Here's the drawing with two shaded views (mm, measured from the low corner). I have some questions. A direction names the side the tool comes from. Coordinates: 2 decimals unless noted, no trailing zeros. Write each loop counter-clockwise with the first axis right and the second up, starting at its lowest first coordinate (ties: lowest second). Pieces come first, ordered by that corner, then holes.
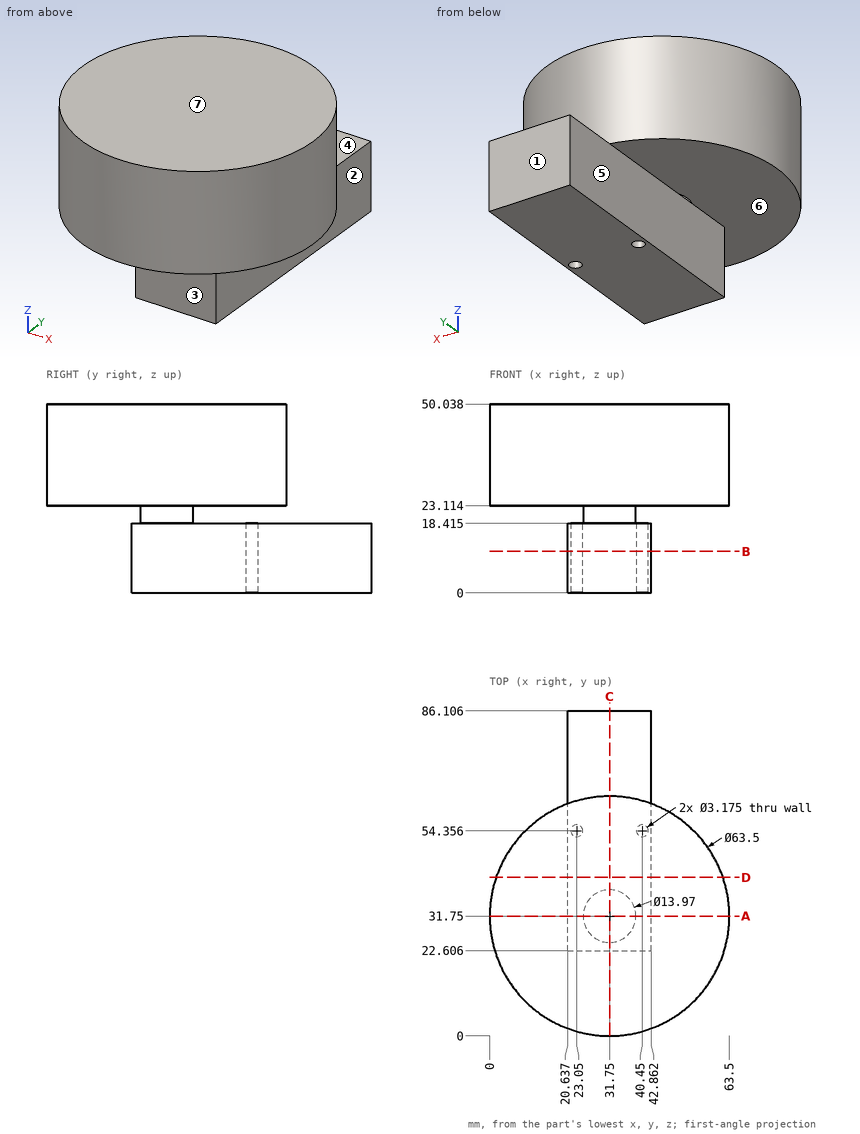
Item 1: I want a section at A-A, the plane y = 31.75. List the corners of the cut face in (x, z) for me (1 decimal), then the cut area to 3 significant figures.
Item 2: If I drill on line 1 along X through (y, z) = (54.5, 17); line 2 along Z through (x, y) = (29, 57) (1 decimal); line 3 along Z through (x, y) = (33, 66) (1 decimal), over which ranges is the centre line in solid material (lowest first)?
Item 3: Will these pins go through, and if not, where does the flat tip stop? pin 1 Ø4 at (x, z) = (54.5, 24.5) entering from -Y; pin 2 Ø9 at (y, z) = (54, 5.5) entering from +X; pin 3 Ø5.5 at (y, z) = (59, 7.5) entering from -X.
Item 4: Which directions (+Z, -Z, +X, -X, +Y, -Y) give clear straight access to the entire face, cutting with the end or side of a thin tool? Please do the marked faces 1, 2 and 3.
Item 5: I want a section at C-C, the plane x = 31.75. List the corners of the cut face in (y, z) for me (1 decimal).
Item 6: I want a section at B-B, the plane z = 11. Count the separate pieces of the cut face and the enclosed holes in it, then the cut area to 3 significant figures.
Item 7: If we mould it in two halves opening along Z, with no side actions, what happens to the marked faces 4, 5, 6 and 7? For each: released by +Z, released by -Z, zero draft, split by the parting line, or undercut.
Item 8: I want a section at D-D, the plane y = 42. List the corners of the cut face in (x, z) for me (1 decimal).
Taken from the geometry:
1. outline: (0, 23.1) - (24.8, 23.1) - (24.8, 18.4) - (20.6, 18.4) - (20.6, 0) - (42.9, 0) - (42.9, 18.4) - (38.7, 18.4) - (38.7, 23.1) - (63.5, 23.1) - (63.5, 50) - (0, 50) - close
1. area: 2,180 mm2
2. line 1: x = 20.64 to 21.47, 24.63 to 38.87, 42.03 to 42.86
2. line 2: z = 0 to 18.4, 23.1 to 50
2. line 3: z = 0 to 18.4
3. pin 1: stops at y = 7.72
3. pin 2: stops at x = 42.86
3. pin 3: stops at x = 20.64
4. face 1: +Z, -Z, +X, -X, +Y
4. face 2: -Z, +X, +Y, -Y
4. face 3: -Z, +X, -X, -Y
5. outline: (0, 23.1) - (24.8, 23.1) - (24.8, 18.4) - (22.6, 18.4) - (22.6, 0) - (86.1, 0) - (86.1, 18.4) - (38.7, 18.4) - (38.7, 23.1) - (63.5, 23.1) - (63.5, 50) - (0, 50) - close
6. separate pieces: 1
6. enclosed holes: 2
6. area: 1,400 mm2
7. face 4: undercut
7. face 5: zero draft
7. face 6: undercut
7. face 7: released by +Z
8. outline: (1.7, 23.1) - (61.8, 23.1) - (61.8, 50) - (1.7, 50) - close; (20.6, 0) - (42.9, 0) - (42.9, 18.4) - (20.6, 18.4) - close
